from build123d import *

# Parameters (mm, degrees)
SKETCH1_W           = 32
SKETCH1_H           = 7
BOSS_EXTRUDE1_DEPTH = 1
SKETCH2_R           = 2.25
BOSS_EXTRUDE2_DEPTH = 4
FILLET1_R           = 0.5


with BuildPart() as part:
    # Sketch1 → Boss-Extrude1 (new body)
    with BuildSketch(Plane(origin=(0, 0, 0), x_dir=(1, 0, 0), z_dir=(0, 1, 0))):
        Rectangle(SKETCH1_W, SKETCH1_H)
    extrude(amount=BOSS_EXTRUDE1_DEPTH)

    # Sketch2 → Boss-Extrude2 (add)
    with BuildSketch(Plane(origin=(0, 1, 0), x_dir=(1, 0, 0), z_dir=(0, 1, 0))):
        with Locations((-13, 0)):
            Circle(SKETCH2_R)
        with Locations((-5, 0)):
            Circle(SKETCH2_R)
        with Locations((5, 0)):
            Circle(SKETCH2_R)
        with Locations((13, 0)):
            Circle(SKETCH2_R)
    extrude(amount=BOSS_EXTRUDE2_DEPTH)

    # Fillet1
    fillet1_edges = [part.edges().sort_by_distance(p)[0] for p in [
        (-15.25, 5, 0),
        (-7.25, 5, 0),
        (2.75, 5, 0),
        (10.75, 5, 0),
    ]]
    fillet(fillet1_edges, radius=FILLET1_R)


solid = part.part
Could you check a few things on this model? Use its own coordinates, in mm. A direction names the side the tool comes from. Round coordinates to 2 decimals unless told otherwise and drop trailing zeros. Write each loop counter-clockwise with the first axis right and the second up, starting at its lowest first coordinate (ties: lowest second). Pieces come first, ordered by that corner, then holes. Notation, with made-up numbers: (19.5, -9) - (72.5, -9) arc R18 ccw to (72.5, 11) - close; hole circle Ø6 at (-1.75, -34.75). An arc over 180 degrees is marked (long way). Put each result on its own line as item: value. Start each with the question number.
(1) Thinking about a two-plate mould opening in X: for faces 3 (the flat face through (-16, 0.5, 0)), 4 (the flat face through (16, 0.5, 0)), 5 (the flat face through (0, 1, 0)), which applies, released by +X, released by -X, zero draft, split by the parting line, or undercut?
(2) For faces 1 (the cylindrical face through (7.146, 2.726, -0.676)), 2 (the flat face through (0, 0, 0)), which set-ups out of +Z, -Z, +X, -X, +Y, -Y let a thin tool reach every point of the face, with its end or its side?
(3) I want a section at B-B, the plane y = 2.3. Please give me the cut outline in (x, z).
(4) I need wall thicknesses on probe 1 along X at (y, z) = (2.75, -0.25); probe 2 along X at (y, z) = (4.6, -1); probe 3 along Y at (x, z) = (-9.5, -0.75). Which ranges of each line are inside material? Lowest first, please.
(5) I want a section at A-A, the plane x = 5. Please give me the cut outline in (y, z), plus the area to 3 significant figures.
Here are the results:
1. face 3: released by -X
1. face 4: released by +X
1. face 5: undercut
2. face 1: +Y
2. face 2: +Z, -Z, +X, -X, -Y
3. outline: circle Ø4.5 at (-13, 0); circle Ø4.5 at (-5, 0); circle Ø4.5 at (5, 0); circle Ø4.5 at (13, 0)
4. probe 1: x = -15.24 to -10.76, -7.24 to -2.76, 2.76 to 7.24, 10.76 to 15.24
4. probe 2: x = -15 to -11, -7 to -3, 3 to 7, 11 to 15
4. probe 3: y = 0 to 1
5. outline: (0, -3.5) - (1, -3.5) - (1, -2.25) - (4.5, -2.25) arc R0.5 ccw to (5, -1.75) - (5, 1.75) arc R0.5 ccw to (4.5, 2.25) - (1, 2.25) - (1, 3.5) - (0, 3.5) - close
5. area: 24.9 mm^2
